The listing builds one solid part. Answer for the finished solid, in the listing's coordinates (mm). Face numbers are marked on the shaded views. A direction names the side the tool comes from. Give positions to 0.01 mm unless a question says otherwise; leave off trailing zeros. Write each loop counter-clockwise with the first axis right and the second up, starting at its lowest first coordinate (ties: lowest second). Pieces come first, ordered by that corner, then holes. Notation, with made-up numbers: (-35.75, 89) -> (4.25, 89) arc R26 cw to (4.25, 113) -> close; hole circle Ø7 at (71, 18). An arc over 180 degrees is marked (long way). Write each question's results on one line, items separated by ' | '. Start each with the question number.
from build123d import *

# Parameters (mm, degrees)
SKETCH_W        = 38
SKETCH_H        = 6.2
SKETCH_R        = 1.5
PAD_DEPTH       = 3
PAD001_DEPTH    = 3.5
PAD002_DEPTH    = 8
SKETCH003_R     = 1.5
POCKET_DEPTH    = 3.101
SKETCH004_W     = 3.1
SKETCH004_H     = 8
PAD003_DEPTH    = 10
SKETCH005_W     = 3.1
SKETCH005_H     = 8
PAD004_DEPTH    = 10
SKETCH006_R     = 1.5
POCKET001_DEPTH = 3.101
CHAMFER_SIZE    = 5
CHAMFER001_SIZE = 3
CHAMFER002_SIZE = 3


with BuildPart() as part:
    # Sketch → Pad (new body)
    with BuildSketch(Plane.XZ):
        with Locations((0, 3.1)):
            Rectangle(SKETCH_W, SKETCH_H)
        with Locations((-14, 3.75)):
            Circle(SKETCH_R, mode=Mode.SUBTRACT)
        with Locations((14, 3.75)):
            Circle(SKETCH_R, mode=Mode.SUBTRACT)
    extrude(amount=PAD_DEPTH)

    # Sketch001 (on Face8 of Pad) → Pad001 (join)
    with BuildSketch(Plane.XZ.offset(3)):
        with BuildLine():
            ThreePointArc((-15.731329, 6.2), (-14, 0.75), (-12.268671, 6.2))
            Line((-12.268671, 6.2), (12.268671, 6.2))
            ThreePointArc((12.268671, 6.2), (14, 0.75), (15.731329, 6.2))
            Line((15.731329, 6.2), (19, 6.2))
            Line((19, 6.2), (19, 0))
            Line((19, 0), (-19, 0))
            Line((-19, 0), (-19, 6.2))
            Line((-19, 6.2), (-15.731329, 6.2))
        make_face()
    extrude(amount=PAD001_DEPTH)

    # Sketch002 (on Face7 of Pad001) → Pad002 (join)
    with BuildSketch(Plane.XZ.offset(6.5)):
        with BuildLine():
            Line((-19, 0), (-19, 3.1))
            Line((-19, 3.1), (-16.928737, 3.1))
            ThreePointArc((-16.928737, 3.1), (-14, 0.75), (-11.071263, 3.1))
            Line((-11.071263, 3.1), (11.071263, 3.1))
            ThreePointArc((11.071263, 3.1), (14, 0.75), (16.928737, 3.1))
            Line((19, 3.1), (16.928737, 3.1))
            Line((19, 0), (19, 3.1))
            Line((-19, 0), (19, 0))
        make_face()
    extrude(amount=PAD002_DEPTH)

    # Sketch003 (on Face13 of Pad002) → Pocket (cut, through all)
    with BuildSketch(Plane(origin=(0, 0, 3.1), x_dir=(-1, 0, 0), z_dir=(0, 0, 1))):
        with Locations((0, 10.5)):
            Circle(SKETCH003_R)
    extrude(amount=-POCKET_DEPTH, mode=Mode.SUBTRACT)

    # Sketch004 (on Face4 of Pocket) → Pad003 (join)
    with BuildSketch(Plane(origin=(19, 0, 0), x_dir=(0, 0, 1), z_dir=(1, 0, 0))):
        with Locations((1.55, 10.5)):
            Rectangle(SKETCH004_W, SKETCH004_H)
    extrude(amount=PAD003_DEPTH)

    # Sketch005 (on Face2 of Pad003) → Pad004 (join)
    with BuildSketch(Plane(origin=(-19, 0, 0), x_dir=(0, 0, -1), z_dir=(-1, 0, 0))):
        with Locations((-1.55, 10.5)):
            Rectangle(SKETCH005_W, SKETCH005_H)
    extrude(amount=PAD004_DEPTH)

    # Sketch006 (on Face23 of Pad004) → Pocket001 (cut, through all)
    with BuildSketch(Plane(origin=(0, 0, 3.1), x_dir=(-1, 0, 0), z_dir=(0, 0, 1))):
        with Locations((-23, 10.5)):
            Circle(SKETCH006_R)
        with Locations((23, 10.5)):
            Circle(SKETCH006_R)
    extrude(amount=-POCKET001_DEPTH, mode=Mode.SUBTRACT)

    # Chamfer
    chamfer_edges = [part.edges().sort_by_distance(p)[0] for p in [
        (-19, -6.5, 1.55),
        (19, -6.5, 1.55),
    ]]
    chamfer(chamfer_edges, length=CHAMFER_SIZE)

    # Chamfer001
    chamfer001_edges = [part.edges().sort_by_distance(p)[0] for p in [
        (-29, -6.5, 1.55),
        (29, -6.5, 1.55),
        (-29, -14.5, 1.55),
        (29, -14.5, 1.55),
    ]]
    chamfer(chamfer001_edges, length=CHAMFER001_SIZE)

    # Chamfer002
    chamfer002_edges = [part.edges().sort_by_distance(p)[0] for p in [
        (-12.268671, -4.75, 6.2),
        (-15.731329, -4.75, 6.2),
        (12.268671, -4.75, 6.2),
        (15.731329, -4.75, 6.2),
    ]]
    chamfer(chamfer002_edges, length=CHAMFER002_SIZE)


solid = part.part
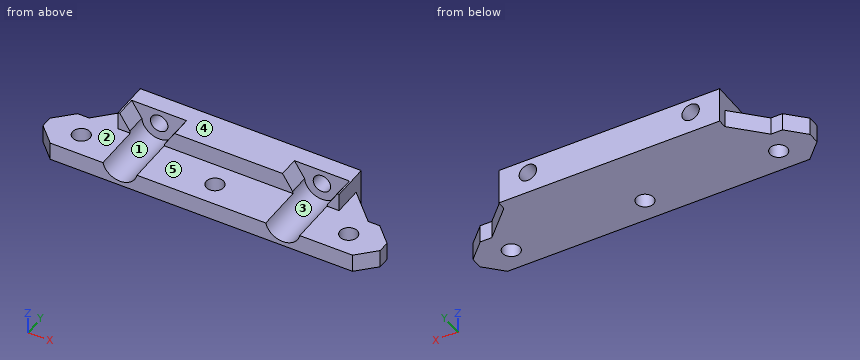
1. Each of these flat-tipped pins is pushed along its axis until it touches: pin 1 Ø3.5 at (x, y) = (-21, -8.5) entering from +Z; pin 2 Ø0.6 at (x, z) = (-18.5, 4) entering from -Y; pin 3 Ø0.6 at (x, z) = (-25, 1.5) entering from +Y; pin 4 Ø2.5 at (x, z) = (-14, 3.75) entering from -Y. Where does it stop, or does it pass through?
2. The mould has two halves that part along X. Classify the marked faces 1 and 2: pulls with the +X half, pulls with the -X half, needs draft (parallel to the pull), parting line crosses it, or undercut.
3. Section C-C (x = 14) is taken. Write down the section's boundary in (y, z).
4. Consider probe 1 along Y at (x, z) = (0, 2.15); probe 2 along X at (y, z) = (-2.75, 3); probe 3 along X at (y, z) = (-3.25, 5.75). Determine where each line is inside the solid, lowest interval first. Write a range as [from, to].
5. Section A-A (x = 0) is taken. Write down the section's boundary in (y, z), then the cut area to 3 significant figures.
6. Section D-D (z = 1.5) is taken. Write down the section's boundary in (x, y).
7. Section B-B (y = -8) is taken. Write down the section's boundary in (x, z).
8. A tool of negligible diameter and unlimited length cuts with its end or side. For the marked faces 3, 4 and 5, from which of +Z, -Z, +X, -X, +Y, -Y can it reach the whole face along a straight path? Write none if from no direction.
Results:
1) pin 1: stops at z = 3.1 | pin 2: stops at y = -6.5 | pin 3: stops at y = -6.5 | pin 4: passes through
2) face 1: undercut | face 2: needs draft
3) outline: (-14.5, 0) -> (0, 0) -> (0, 2.25) -> (-3, 2.25) -> (-3, 0.75) -> (-14.5, 0.75) -> close; (-3, 5.25) -> (0, 5.25) -> (0, 6.2) -> (-3, 6.2) -> close
4) probe 1: y = [-14.5, -12], [-9, 0] | probe 2: x = [-20.25, -15.3], [-12.7, 12.7], [15.3, 20.25] | probe 3: x = [-19, -18.44], [-9.56, 9.56], [18.44, 19]
5) outline: (-14.5, 0) -> (-12, 0) -> (-12, 3.1) -> (-14.5, 3.1) -> close; (-9, 0) -> (0, 0) -> (0, 6.2) -> (-6.5, 6.2) -> (-6.5, 3.1) -> (-9, 3.1) -> close | area: 55.8 mm²
6) outline: (-29, -11.5) -> (-26, -14.5) -> (-15.98, -14.5) -> (-15.98, -3) -> (-12.02, -3) -> (-12.02, -14.5) -> (12.02, -14.5) -> (12.02, -3) -> (15.98, -3) -> (15.98, -14.5) -> (26, -14.5) -> (29, -11.5) -> (29, -9.5) -> (26, -6.5) -> (24, -6.5) -> (19, -1.5) -> (19, 0) -> (-19, 0) -> (-19, -1.5) -> (-24, -6.5) -> (-26, -6.5) -> (-29, -9.5) -> close; hole circle Ø3 at (-23, -10.5); hole circle Ø3 at (0, -10.5); hole circle Ø3 at (23, -10.5)
7) outline: (-27.5, 0) -> (27.5, 0) -> (27.5, 3.1) -> (16.93, 3.1) arc R3 cw to (11.07, 3.1) -> (-11.07, 3.1) arc R3 cw to (-16.93, 3.1) -> (-27.5, 3.1) -> close
8) face 3: +Z, -Y | face 4: +Z, +X, -X, +Y, -Y | face 5: +Z, +X, -X, -Y
